Build history of the part. All positions in model axes, mm. A direction names the side the tool comes from. Round coordinates to 2 decimals unless told otherwise and drop trailing zeros. Loops run counter-clockwise (first coordinate to the right, second up) from the corner with the lowest first, then second, coordinate; pieces in that order, holes last.
from build123d import *

# Parameters (mm, degrees)
SKETCH_R           = 28.5
PAD_DEPTH          = 21.5
SKETCH001_R        = 7.5
PAD001_DEPTH       = 3.3
SKETCH002_R        = 1.4
POCKET_DEPTH       = 22
POCKET001_DEPTH    = 190.178681
POLARPATTERN_COUNT = 5
CHAMFER_SIZE       = 1
CHAMFER001_SIZE    = 1
CHAMFER002_SIZE    = 1
CHAMFER003_SIZE    = 1


with BuildPart() as part:
    # Sketch → Pad (new body)
    with BuildSketch(Plane.XY):
        Circle(SKETCH_R)
    extrude(amount=PAD_DEPTH)

    # Sketch001 (on Face3 of Pad) → Pad001 (join)
    with BuildSketch(Plane.XY.offset(21.5)):
        Circle(SKETCH001_R)
    extrude(amount=PAD001_DEPTH)

    # Sketch002 (on Face5 of Pad001) → Pocket (cut)
    with BuildSketch(Plane.XY.offset(24.8)):
        Circle(SKETCH002_R)
    extrude(amount=-POCKET_DEPTH, mode=Mode.SUBTRACT)

    # Sketch003 (on Face3 of Pocket) → Pocket001 (cut, through all)
    with BuildSketch(Plane.XY.offset(21.5)):
        with BuildLine():
            Line((-6.437201, 6.159132), (-16.552795, 15.837703))
            ThreePointArc((0, 22.909122), (-9, 21.067223), (-16.552795, 15.837703))
            Line((0, 22.909122), (0, 8.909122))
            ThreePointArc((0, 8.909122), (-3.5, 8.19283), (-6.437201, 6.159132))
        make_face()
    pocket001 = extrude(amount=-POCKET001_DEPTH, mode=Mode.SUBTRACT)

    # PolarPattern: Pocket001 ×5 about axis
    polarpattern_axis = Axis((0, 0, 21.5), (0, 0, 1))
    for i in range(1, POLARPATTERN_COUNT):
        add(pocket001.rotate(polarpattern_axis, i * 360 / POLARPATTERN_COUNT), mode=Mode.SUBTRACT)

    # Chamfer
    chamfer_edges = [part.edges().sort_by_distance(p)[0] for p in [
        (-1.4, 0, 24.8),
    ]]
    chamfer(chamfer_edges, length=CHAMFER_SIZE)

    # Chamfer001
    chamfer001_edges = [part.edges().sort_by_distance(p)[0] for p in [
        (-28.5, 0, 21.5),
    ]]
    chamfer(chamfer001_edges, length=CHAMFER001_SIZE)

    # Chamfer002
    chamfer002_edges = [part.edges().sort_by_distance(p)[0] for p in [
        (-28.5, 0, 0),
    ]]
    chamfer(chamfer002_edges, length=CHAMFER002_SIZE)

    # Chamfer003
    chamfer003_edges = [part.edges().sort_by_distance(p)[0] for p in [
        (-7.5, 0, 24.8),
    ]]
    chamfer(chamfer003_edges, length=CHAMFER003_SIZE)


solid = part.part
(1) Slice it at A-A on y = 0. List the corners of the cut face in (x, z).
Responses:
outline: (-28.5, 1) - (-27.5, 0) - (-22.91, 0) - (-22.91, 21.5) - (-27.5, 21.5) - (-28.5, 20.5) - close; (-8.91, 0) - (27.5, 0) - (28.5, 1) - (28.5, 20.5) - (27.5, 21.5) - (7.5, 21.5) - (7.5, 23.8) - (6.5, 24.8) - (2.4, 24.8) - (1.4, 23.8) - (1.4, 2.8) - (-1.4, 2.8) - (-1.4, 23.8) - (-2.4, 24.8) - (-6.5, 24.8) - (-7.5, 23.8) - (-7.5, 21.5) - (-8.91, 21.5) - close
(2) Probe line 1 (X direction, y = -11, z = 19); line 2 (Y direction, x = -1.5, z = 17); line 3 (Y direction, x = 17.5, z = 17.25). List the from-to ranges inside material, lowest first.
Responses:
line 1: x = -26.29 to -7.99, 1.99 to 7.99, 20.1 to 26.29
line 2: y = -28.46 to -22.86, -8.78 to 8.78, 22.86 to 28.46
line 3: y = -22.49 to -14.78, -2.38 to 5.69, 14.78 to 22.49
(3) Pull direction X, two halves, no side cores. Call faces 1 (the face through (-11.424, 10.931, 10.901)), 2 (the face through (3, 0, 24.8)): +X half, -X half, draft (parallel to the pull), parting line (faces both ways), or undercut.
Responses:
face 1: undercut
face 2: draft
(4) Which spindle directions (+Z, -Z, +X, -X, +Y, -Y) get a long thin tool onto all of the face, cutting with end or side? Do faces 3 (the face through (6, -6, 21.5)), 4 (the face through (-5.228, -22.305, 10.901)), 5 (the face through (0, 0, 0)). Say none if no direction does.
Responses:
face 3: +Z
face 4: +Z, -Z
face 5: -Z, +X, -X, +Y, -Y
(5) Pin check, flat tips, straight feed: P1, Ø5, axis at y = -2.5, z = 12.5, coming from the +X side; P2, Ø2, axis at x = 19.5, z = 13.5, coming from the +Y side; P3, Ø1.5, axis at x = -13.5, z = 7.5, coming from the -Y side; P4, Ø6, axis at y = 5, z = 14, coming from the +X side. Stop position of each tip, or through.
Responses:
P1: stops at x = 28.5
P2: stops at y = 21.68
P3: stops at y = -25.49
P4: stops at x = 28.43
(6) Slice it at D-D on x = 15.5. Count the separate pieces of the cut face and the enclosed holes in it, plus the area to 3 significant figures.
Responses:
separate pieces: 3
enclosed holes: 0
area: 454 mm2
(7) Slice it at B-B on z = 13.25. List the corners of the cut face in (x, y), plus the area to 3 significant figures.
Responses:
outline: circle Ø57 at (0, 0); hole (-21.79, 7.08) arc R22.91 ccw to (-20.18, -10.85) - (-7.85, -4.22) arc R8.91 cw to (-8.47, 2.75) - close; hole (-16.55, 15.84) - (-6.44, 6.16) arc R8.91 cw to (0, 8.91) - (0, 22.91) arc R22.91 ccw to start; hole (-13.47, -18.53) arc R22.91 ccw to (4.08, -22.54) - (1.59, -8.77) arc R8.91 cw to (-5.24, -7.21) - close; hole circle Ø2.8 at (0, 0); hole (3.87, 8.03) arc R8.91 cw to (8.47, 2.75) - (21.79, 7.08) arc R22.91 ccw to (9.95, 20.64) - close; hole (5.24, -7.21) - (13.47, -18.53) arc R22.91 ccw to (22.7, -3.08) - (8.83, -1.2) arc R8.91 cw to start
area: 1,650 mm2
(8) Slice it at C-C on z = 2. List the corners of the cut face in (x, y), plus the area to 3 significant figures.
Responses:
outline: circle Ø57 at (0, 0); hole (-21.79, 7.08) arc R22.91 ccw to (-20.18, -10.85) - (-7.85, -4.22) arc R8.91 cw to (-8.47, 2.75) - close; hole (-16.55, 15.84) - (-6.44, 6.16) arc R8.91 cw to (0, 8.91) - (0, 22.91) arc R22.91 ccw to start; hole (-13.47, -18.53) arc R22.91 ccw to (4.08, -22.54) - (1.59, -8.77) arc R8.91 cw to (-5.24, -7.21) - close; hole (3.87, 8.03) arc R8.91 cw to (8.47, 2.75) - (21.79, 7.08) arc R22.91 ccw to (9.95, 20.64) - close; hole (5.24, -7.21) - (13.47, -18.53) arc R22.91 ccw to (22.7, -3.08) - (8.83, -1.2) arc R8.91 cw to start
area: 1,650 mm2
